Answer from the drawing. Dimensions are ordinates in mm from the lowest x, y and z of the part. Give positions to 0.01 mm unless a question says otherwise; leave off trailing zeros. Write each loop counter-clockwise with the first axis right and the second up, starting at its lowest first coordinate (ties: lowest second). Pieces come first, ordered by that corner, then holes.
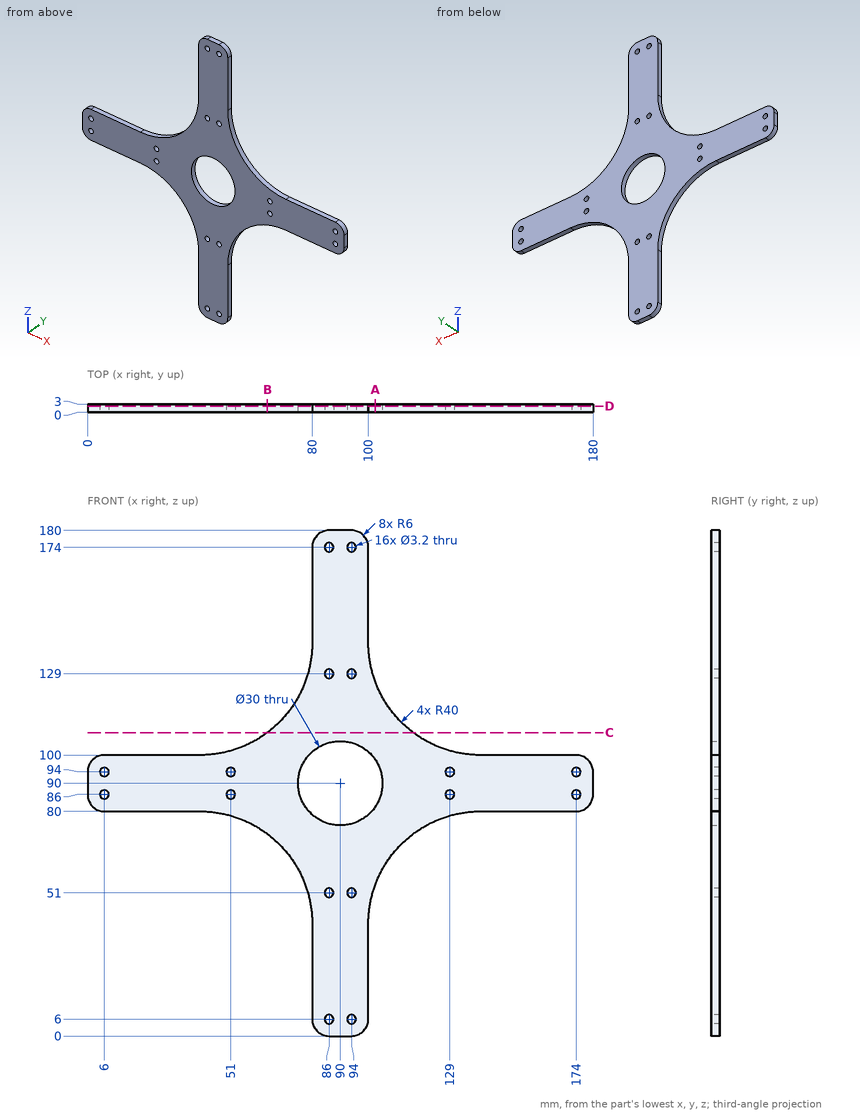
Item 1: Find the intervals of material crossed by line 1 along X through (y, z) = (0.95, 90); line 2 along X through (y, z) = (1.05, 94); line 3 along X through (y, z) = (1.75, 51), in increasing order.
Result set:
line 1: x = 0 to 75, 105 to 180
line 2: x = 0 to 4.4, 7.6 to 49.4, 52.6 to 75.54, 104.46 to 127.4, 130.6 to 172.4, 175.6 to 180
line 3: x = 78.46 to 84.4, 87.6 to 92.4, 95.6 to 101.54
Item 2: Section B-B (x = 64) is taken. Write down the section's boundary in (y, z), and give its area (3 significant figures).
Result set:
outline: (0, 72) - (3, 72) - (3, 108) - (0, 108) - close
area: 108 mm2
Item 3: Section C-C (z = 108) is taken. Write down the section's boundary in (x, y).
Result set:
outline: (64, 0) - (116, 0) - (116, 3) - (64, 3) - close
Item 4: Section D-D (y = 2.2) is taken. Give the number of separate pieces and of enclosed holes in the cut face, and give its area (3 significant figures).
Result set:
separate pieces: 1
enclosed holes: 17
area: 7,280 mm2
Item 5: Section A-A (x = 102.5) is taken. Write down the section's boundary in (y, z).
Result set:
outline: (0, 53.92) - (3, 53.92) - (3, 81.71) - (0, 81.71) - close; (0, 98.29) - (3, 98.29) - (3, 126.08) - (0, 126.08) - close
Item 6: Each of these flat-tipped pins is pushed along its axis until it touches: pin 1 Ø1 at (x, y) = (126.5, 2) entering from +Z; pin 2 Ø1.5 at (x, z) = (69, 69.5) entering from -Y; pin 3 Ø0.9 at (y, z) = (2, 152) entering from -X; pin 4 Ø1.5 at (x, y) = (25, 1) entering from -Z. Where does it stop, or does it pass through?
Result set:
pin 1: stops at z = 102.53
pin 2: stops at y = 0
pin 3: stops at x = 80
pin 4: stops at z = 80
